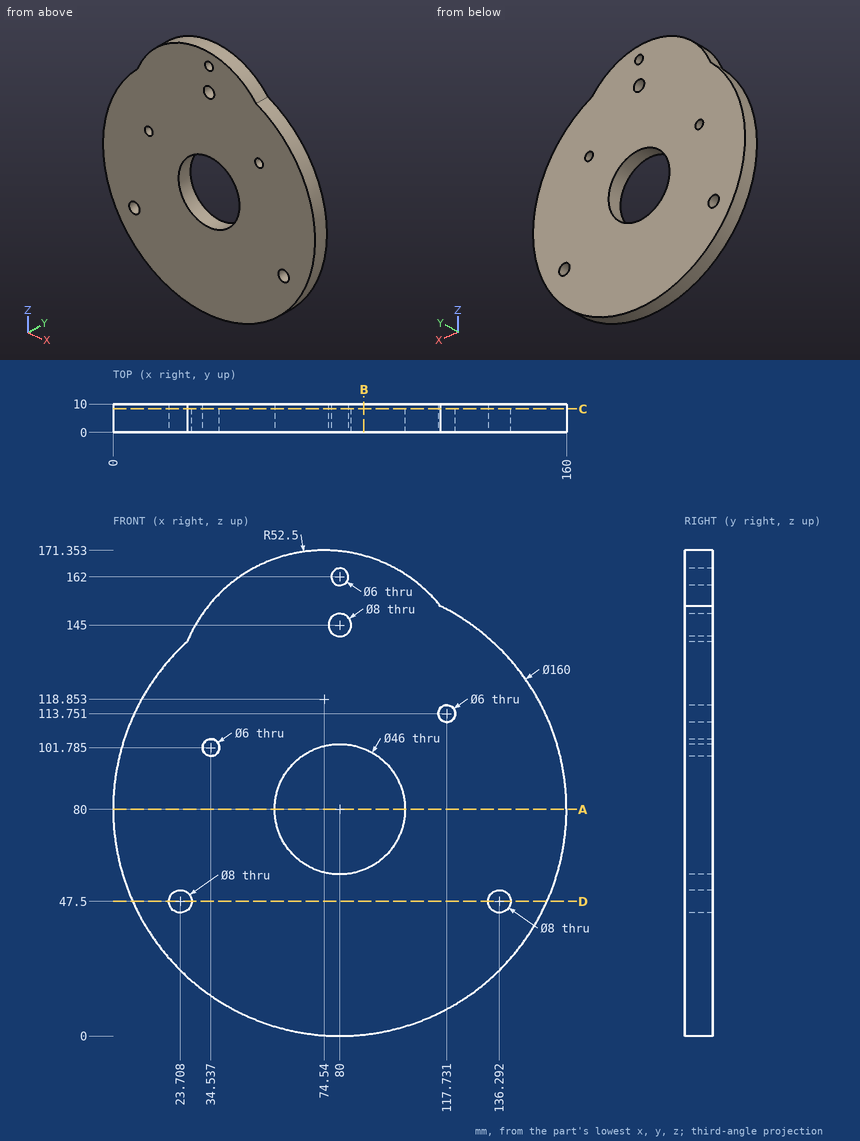
Study the drawing (mm; zero at the part's minimum x, y, z) and answer. Round coordinates to 2 decimals unless told otherwise and drop trailing zeros. Order: outer loops, then holes, each group sorted by start corner. A loop starts at its lowest first (then second) coordinate and runs counter-clockwise, first axis right, second up. Notation, with made-up numbers: (72.25, 41) - (76.25, 41) arc R23 cw to (76.25, 71) - close; hole circle Ø11 at (23, 82). An arc over 180 degrees is marked (long way). Use one line per item in the form item = value. Start each with the question number.
(1) The part is cut by section C-C (y = 8.25). Give the vertices of the cut face in (x, z) (1 decimal).
(2) The part is cut by section D-D (z = 47.5). Give the vertices of the cut face in (x, y).
(3) The part is cut by section A-A (z = 80). Give the vertices of the cut face in (x, y).
(4) Flat-ended cylindrical pins translate along their axes: pin 1 Ø1 at (x, y) = (76.5, 6.5) entering from +Z; pin 2 Ø2 at (x, y) = (70, 1.5) entering from +Z; pin 3 Ø6 at (x, y) = (94, 3) entering from +Z (1 decimal); pin 4 Ø3.5 at (x, z) = (34.54, 101.79) entering from +Y. Find the tip coordinate at first contact, or state that the pin passes through.
(5) The part is cut by section B-B (x = 88.5). Give the vertices of the cut face in (y, z).
(6) Find the intervals of material crossed by line 1 along X through (y, z) = (4.5, 47.5); line 2 along X through (y, z) = (2.75, 80); line 3 along Z through (x, y) = (80, 4.5), in increasing order. Write a range as from..to.
Checked values:
q1.outline = (26.1, 139.1) arc R80 ccw (long way) to (115.5, 151.7) arc R52.5 ccw to start; hole circle Ø8 at (23.7, 47.5); hole circle Ø6 at (34.5, 101.8); hole circle Ø46 at (80, 80); hole circle Ø8 at (80, 145); hole circle Ø6 at (80, 162); hole circle Ø6 at (117.7, 113.8); hole circle Ø8 at (136.3, 47.5)
q2.outline = (6.9, 0) - (19.71, 0) - (19.71, 10) - (6.9, 10) - close; (27.71, 0) - (132.29, 0) - (132.29, 10) - (27.71, 10) - close; (140.29, 0) - (153.1, 0) - (153.1, 10) - (140.29, 10) - close
q3.outline = (0, 0) - (57, 0) - (57, 10) - (0, 10) - close; (103, 0) - (160, 0) - (160, 10) - (103, 10) - close
q4.pin_1 = 171.33
q4.pin_2 = 171.23
q4.pin_3 = 168.7
q4.pin_4 = through
q5.outline = (0, 0.45) - (10, 0.45) - (10, 58.63) - (0, 58.63) - close; (0, 101.37) - (10, 101.37) - (10, 169.46) - (0, 169.46) - close
q6.line_1 = 6.9..19.71, 27.71..132.29, 140.29..153.1
q6.line_2 = 0..57, 103..160
q6.line_3 = 0..57, 103..141, 149..159, 165..171.07
